from build123d import *

# Parameters (mm, degrees)
IZIM1_W                     = 36
IZIM1_H                     = 36
IZIM1_R                     = 8
Y_KSEKLIK_EKSTR_ZYON1_DEPTH = 50
IZIM2_W                     = 36
IZIM2_H                     = 5
KES_EKSTR_ZYON1_DEPTH       = 50
IZIM3_W                     = 36
IZIM3_H                     = 3
KES_EKSTR_ZYON2_DEPTH       = 50
KES_EKSTR_ZYON3_DEPTH       = 50
M4_BO_LUKLU_DELIK1_D        = 4.5
KES_EKSTR_ZYON6_START       = -50
KES_EKSTR_ZYON6_DEPTH       = 50


# Read off the part's stored shape, not the designer's step: Kes-Ekstrüzyon6
with BuildPart() as part:
    # Çizim1 → Yükseklik-Ekstrüzyon1 (new body)
    with BuildSketch(Plane.XY):
        Rectangle(IZIM1_W, IZIM1_H)
        Circle(IZIM1_R, mode=Mode.SUBTRACT)
    extrude(amount=Y_KSEKLIK_EKSTR_ZYON1_DEPTH)

    # Çizim2 → Kes-Ekstrüzyon1 (cut)
    with BuildSketch(Plane.XY.offset(50)):
        with Locations((0, 15.5)):
            Rectangle(IZIM2_W, IZIM2_H)
    extrude(amount=-KES_EKSTR_ZYON1_DEPTH, mode=Mode.SUBTRACT)

    # Çizim3 → Kes-Ekstrüzyon2 (cut)
    with BuildSketch(Plane.XY.offset(50)):
        with Locations((0, -16.5)):
            Rectangle(IZIM3_W, IZIM3_H)
    extrude(amount=-KES_EKSTR_ZYON2_DEPTH, mode=Mode.SUBTRACT)

    # Çizim4 → Kes-Ekstrüzyon3 (cut)
    with BuildSketch(Plane.XY.offset(50)):
        Polygon((-6.350852961, -11), (-9.526279442, -5.5), (-18, -5.5), (-18, -15), (18, -15), (18, -5.5), (9.526279442, -5.5), (6.350852961, -11), align=None)
    extrude(amount=-KES_EKSTR_ZYON3_DEPTH, mode=Mode.SUBTRACT)

    # M4 Boşluklu Delik1 (through all)
    with Locations(Plane(origin=(0, -5.5, 0), x_dir=(-1, 0, 0), z_dir=(0, -1, 0))):
        with Locations((-13.718329125, -40), (-13.718329125, -10), (12.810498521, -10), (12.810498521, -40)):
            Hole(M4_BO_LUKLU_DELIK1_D / 2)

    # Kes-Ekstrüzyon6 outline → Kes-Ekstrüzyon6 (cut)
    with BuildSketch(Plane.XY.offset(50).offset(KES_EKSTR_ZYON6_START)):
        with BuildLine():
            Line((18, -5.5), (18, 3.75))
            Line((18, 3.75), (7.066647013, 3.75))
            ThreePointArc((7.066647013, 3.75), (0, -8), (-7.066647013, 3.75))
            Line((-7.066647013, 3.75), (-18, 3.75))
            Line((-18, 3.75), (-18, -5.5))
            Line((-18, -5.5), (-9.526279442, -5.5))
            Line((-9.526279442, -5.5), (-6.350852961, -11))
            Line((-6.350852961, -11), (6.350852961, -11))
            Line((6.350852961, -11), (9.526279442, -5.5))
            Line((9.526279442, -5.5), (18, -5.5))
        make_face()
    extrude(amount=KES_EKSTR_ZYON6_DEPTH, mode=Mode.SUBTRACT)


solid = part.part
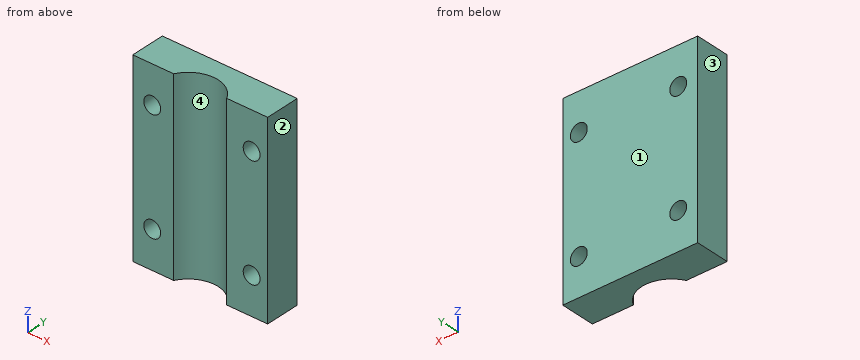
Geometry: final body of the model. Coordinates: model frame, mm. Face numbers are marked on the shaded views. Round coordinates to 2 decimals unless told otherwise and drop trailing zeros. Order: outer loops, then holes, each group sorted by start corner. A loop starts at its lowest first (then second) coordinate and runs counter-clockwise, first axis right, second up. Notation, with made-up numbers: (-1, 83) -> (44, 83) arc R15 cw to (44, 99) -> close; hole circle Ø9 at (89, 72.25). An arc over 180 degrees is marked (long way). Put each result on its own line as item: value. Start each with the question number.
Q1. Section B-B on y = 12.25. Return the cut outline in (x, z).
Q2. Section C-C on z = 10. Return the cut outline in (x, y), and give its area (3 significant figures).
Q3. Pull-direction query (X, two-part tool) for the marked faces 1, 2, 3 and 4; classes: +X half, -X half, draft (parallel to the pull), parting line (faces both ways), or undercut.
Q4. Section A-A on y = 6.5. Return the cut outline in (x, z).
Q5. Line query: probe 1 along X at (y, z) = (11, 40); probe 2 along X at (y, z) = (6.75, 40); probe 3 along X at (y, z) = (10.25, 42). Output: solid intervals per line, ascending.
Q6. Section D-D on x = -13.5. Return the cut outline in (y, z), and give its area (3 significant figures).
Ans:
1. outline: (-18, 0) -> (18, 0) -> (18, 50) -> (-18, 50) -> close; hole circle Ø4.5 at (-12.81, 10); hole circle Ø4.5 at (-12.81, 40); hole circle Ø4.5 at (13.72, 10); hole circle Ø4.5 at (13.72, 40)
2. outline: (-18, 3.75) -> (-15.06, 3.75) -> (-15.06, 13) -> (-18, 13) -> close; (-10.56, 3.75) -> (-7.07, 3.75) arc R8 cw to (7.07, 3.75) -> (11.47, 3.75) -> (11.47, 13) -> (-10.56, 13) -> close; (15.97, 3.75) -> (18, 3.75) -> (18, 13) -> (15.97, 13) -> close
2. area: 207 mm2
3. face 1: draft
3. face 2: +X half
3. face 3: -X half
3. face 4: undercut
4. outline: (-18, 0) -> (-4.66, 0) -> (-4.66, 50) -> (-18, 50) -> close; (4.66, 0) -> (18, 0) -> (18, 50) -> (4.66, 50) -> close; hole circle Ø4.5 at (-12.81, 10); hole circle Ø4.5 at (-12.81, 40); hole circle Ø4.5 at (13.72, 10); hole circle Ø4.5 at (13.72, 40)
5. probe 1: x = -18 to -15.06, -10.56 to 11.47, 15.97 to 18
5. probe 2: x = -18 to -15.06, -10.56 to -4.29, 4.29 to 11.47, 15.97 to 18
5. probe 3: x = -18 to -13.84, -11.78 to 12.69, 14.75 to 18
6. outline: (3.75, 0) -> (13, 0) -> (13, 7.86) -> (3.75, 7.86) -> close; (3.75, 12.14) -> (13, 12.14) -> (13, 37.86) -> (3.75, 37.86) -> close; (3.75, 42.14) -> (13, 42.14) -> (13, 50) -> (3.75, 50) -> close
6. area: 383 mm2
